CAD build for the part. Positions are in the model's coordinates, mm. A direction names the side the tool comes from. Round coordinates to 2 decimals unless told otherwise and drop trailing zeros. Write each loop counter-clockwise with the first axis right and the second up, starting at its lowest first coordinate (ties: lowest second). Pieces come first, ordered by that corner, then holes. Notation, with made-up numbers: (-36.75, 2) - (22.25, 2) arc R13 ccw to (22.25, 11) - close; hole circle Ø7 at (48.5, 10.5). An arc over 180 degrees is marked (long way). Answer in a Markdown table with one row per item.
Autodesk Inventor part; units mm, degrees
ref_plane "YZ Plane" through (0, 0, 0) normal (1, 0, 0) x (0, 1, 0)
ref_plane "XZ Plane" through (0, 0, 0) normal (0, 1, 0) x (-1, 0, 0)
ref_plane "XY Plane" through (0, 0, 0) normal (0, 0, 1) x (1, 0, 0)
sketch "Sketch1" plane through (0, 0, 0) normal (0, 0, 1) x (1, 0, 0)
  line L0 (0, 0) -> (119, 0)
  line L1 (119, 0) -> (119, 80)
  line L2 (119, 80) -> (0, 80)
  line L3 (0, 80) -> (0, 0)
  dimension "d0" = 119
  dimension "d1" = 80
extrude "Extrusion1" add sketch "Sketch1" along normal blind 10
sketch "Sketch2" plane through (0, 0, 10) normal (0, 0, 1) x (1, 0, 0)
  line L0 (-10, 60) -> (0, 60)
  line L1 (0, 60) -> (0, 20)
  line L2 (0, 20) -> (-10, 20)
  line L3 (-10, 20) -> (-10, 60)
  line L4 (0, 80) -> (0, 0)
  circle A0 centre (-5, 40) radius 2.5
  point P0 (0, 40)
  point P1 (0, 40)
  point P2 (0, 40)
  point P3 (0, 40)
  point P4 (-5, 60)
  dimension "d4" = 10
  dimension "d5" = 40
  dimension "d6" = 5
extrude "Extrusion2" add sketch "Sketch2" against normal blind 10
sketch "Sketch3" plane through (0, 0, 10) normal (0, 0, 1) x (1, 0, 0)
  circle A0 centre (9.5, 60) radius 2
  line L0 (0, 80) -> (0, 60)
  line L1 (119, 80) -> (0, 80)
  circle A1 centre (9.5, 20) radius 2
  point P0 (0, 0)
  dimension "d12" = 4
  dimension "d13" = 9.5
  dimension "d14" = 20
  dimension "d15" = 4
  dimension "d16" = 40
extrude "Extrusion3" cut sketch "Sketch3" against normal through all
sketch "Sketch4" plane through (0, 0, 10) normal (0, 0, 1) x (1, 0, 0)
  line L0 (0, 80) -> (0, 60)
  line L1 (0, 20) -> (-10, 20)
  line L2 (0, 60) -> (-10, 60)
  line L3 (-10, 60) -> (-10, 20)
  line L4 (-10, 20) -> (0, 20)
  line L5 (0, 20) -> (0, 60)
  point P0 (0, 0)
extrude "Extrusion4" cut sketch "Sketch4" against normal blind 5
sketch "Sketch5" plane through (0, 0, 10) normal (0, 0, 1) x (1, 0, 0)
  circle A0 centre (59.5, 70.5) radius 2.5
  line L0 (119, 80) -> (0, 80)
  point P0 (0, 0)
  point P1 (59.5, 80)
  dimension "d21" = 5
  dimension "d22" = 9.5
extrude "Extrusion5" cut sketch "Sketch5" against normal through all
properties part number "SP001" material "ABS Plastic"
Q1. Drill centre lines: line 1 (Y direction, x = 9.5, z = 6.5); line 2 (Y direction, x = -5, z = 1.85); line 3 (X direction, y = 9.5, z = 8.25). Where is each one in solid material? Low to high.
Computed:
| item | result |
|---|---|
| line 1 | y = 0 to 18, 22 to 58, 62 to 80 |
| line 2 | y = 20 to 37.5, 42.5 to 60 |
| line 3 | x = 0 to 119 |
Q2. 3-axis set-ups, long thin cutter, end or side, ignore diameter. For faces 5 (the flat face through (-5, 60, 3)), 6 (the flat face through (-8, 40, 5)), 7 (the flat face through (-5, 20, 3)): which of +Z, -Z, +X, -X, +Y, -Y reach the whole face in a straight line?
Computed:
| item | result |
|---|---|
| face 5 | +Z, -Z, -X, +Y |
| face 6 | +Z, -X, +Y, -Y |
| face 7 | +Z, -Z, -X, -Y |
Q3. Flat gauge pins, fed straight in: pin 1 (2.5 mm diameter, centred on x = -6, z = 2, fed in from +Y); pin 2 (2.5 mm diameter, centred on x = -7, z = 2.5, fed in from -Y); pin 3 (3 mm diameter, centred on x = -3, y = 43, fed in from +Z). Where does each tip first touch, or does it go through?
Computed:
| item | result |
|---|---|
| pin 1 | stops at y = 60 |
| pin 2 | stops at y = 20 |
| pin 3 | stops at z = 5 |
Q4. Pull direction Y, two halves, no side cores. Call faces 1 (the cylindrical face through (-5.54, 37.56, 2.54)), 2 (the cylindrical face through (9.24, 61.983, 5.07)), 3 (the flat face through (60, 80, 5)), 4 (the flat face through (119, 39, 5)): released by +Y, released by -Y, zero draft, split by the parting line, or undercut.
Computed:
| item | result |
|---|---|
| face 1 | undercut |
| face 2 | undercut |
| face 3 | released by +Y |
| face 4 | zero draft |
Q5. Saw through at B-B on x = 9.5. List the corners of the cut face in (y, z).
Computed:
| item | result |
|---|---|
| outline | (0, 0) - (18, 0) - (18, 10) - (0, 10) - close; (22, 0) - (58, 0) - (58, 10) - (22, 10) - close; (62, 0) - (80, 0) - (80, 10) - (62, 10) - close |
Q6. Saw through at A-A on y = 70.5. List the corners of the cut face in (x, z).
Computed:
| item | result |
|---|---|
| outline | (0, 0) - (57, 0) - (57, 10) - (0, 10) - close; (62, 0) - (119, 0) - (119, 10) - (62, 10) - close |
Q7. Saw through at C-C on z = 3.5. List the corners of the cut face in (x, y).
Computed:
| item | result |
|---|---|
| outline | (-10, 20) - (0, 20) - (0, 0) - (119, 0) - (119, 80) - (0, 80) - (0, 60) - (-10, 60) - close; hole circle Ø5 at (-5, 40); hole circle Ø4 at (9.5, 20); hole circle Ø4 at (9.5, 60); hole circle Ø5 at (59.5, 70.5) |
Q8. Saw through at D-D on x = 59.5. List the corners of the cut face in (y, z).
Computed:
| item | result |
|---|---|
| outline | (0, 0) - (68, 0) - (68, 10) - (0, 10) - close; (73, 0) - (80, 0) - (80, 10) - (73, 10) - close |
